Input: part model. Units: mm. Frame: model coordinates. Face numbers are marked on the shaded views. Coordinates: 2 decimals unless noted, no trailing zeros. Write each loop counter-clockwise with the first axis right and the second up, starting at its lowest first coordinate (ties: lowest second). Pieces come first, ordered by that corner, then holes. Notation, with made-up numbers: (74, 31) - (128, 31) arc R19 ccw to (128, 41) - close; hole circle Ø7 at (-10, -10.5). An arc over 180 degrees is marked (long way). Use CSV: the item, a comma, the result in double quotes.
```python
from build123d import *

# Parameters (mm, degrees)
SKETCH1_R           = 12.4
BOSS_EXTRUDE1_DEPTH = 59
SKETCH2_R           = 1.5
CUT_EXTRUDE1_DEPTH  = 3.4798
SKETCH4_R           = 4
BOSS_EXTRUDE3_DEPTH = 2.3
SKETCH5_R           = 2
BOSS_EXTRUDE4_DEPTH = 15.5


with BuildPart() as part:
    # Sketch1 → Boss-Extrude1 (new body)
    with BuildSketch(Plane(origin=(0, 0, 0), x_dir=(1, 0, 0), z_dir=(0, 1, 0))):
        with Locations(Location((0, 0, 0), (0, 0, 90))):
            Circle(SKETCH1_R)
    extrude(amount=BOSS_EXTRUDE1_DEPTH)

    # Sketch2 → Cut-Extrude1 (cut)
    with BuildSketch(Plane(origin=(0, 59, 0), x_dir=(1, 0, 0), z_dir=(0, 1, 0))):
        with Locations(Location((0, 8.5, 0), (0, 0, 270))):
            Circle(SKETCH2_R)
        with Locations(Location((0, -8.5, 0), (0, 0, 270))):
            Circle(SKETCH2_R)
    extrude(amount=-CUT_EXTRUDE1_DEPTH, mode=Mode.SUBTRACT)

    # Sketch4 → Boss-Extrude3 (add)
    with BuildSketch(Plane(origin=(0, 59, 0), x_dir=(1, 0, 0), z_dir=(0, 1, 0))):
        with Locations(Location((0, 0, 0), (0, 0, 270))):
            Circle(SKETCH4_R)
    extrude(amount=BOSS_EXTRUDE3_DEPTH)

    # Sketch5 → Boss-Extrude4 (add)
    with BuildSketch(Plane(origin=(0, 61.3, 0), x_dir=(1, 0, 0), z_dir=(0, 1, 0))):
        with Locations(Location((0, 0, 0), (0, 0, 270))):
            Circle(SKETCH5_R)
    extrude(amount=BOSS_EXTRUDE4_DEPTH)


solid = part.part
```
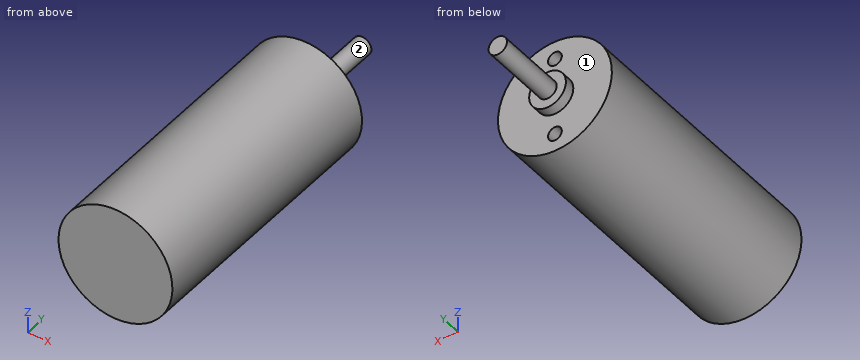
(1) Cut plane B-B on y = 30. Return loops of the section in (x, z), and give its area (3 significant figures).
Check values:
outline,"circle Ø24.8 at (0, 0)"
area,"483 mm^2"
(2) Draft query along Z for the marked faces 1 and 2. Return one class per face: pulls with the +Z half, pulls with the -Z half, needs draft (parallel to the pull), parting line crosses it, or undercut.
Check values:
face 1,"needs draft"
face 2,"parting line crosses it"
(3) Ray query, probe 1 along Y at (x, z) = (8.25, 2); probe 2 along Y at (x, z) = (2.25, 0); probe 3 along X at (y, z) = (20, -5.75). Return the intervals inside material, ascending. Write a range as from..to.
Check values:
probe 1,"0..59"
probe 2,"0..61.3"
probe 3,"-10.99..10.99"
(4) Pin query (flat end, axial travel): pin 1 Ø3 at (x, y) = (7, 55) entering from -Z; pin 2 Ø6 at (x, y) = (-9, 30.5) entering from +Z; pin 3 Ø3.5 at (x, z) = (0.5, -8) entering from +Y. Return the tip coordinate at first contact, or that it passes through.
Check values:
pin 1,"z = -11.11"
pin 2,"z = 10.85"
pin 3,"y = 59"
(5) Cut plane D-D on z = -9. Return loops of the section in (x, y), and give its area (3 significant figures).
Check values:
outline,"(-8.53, 0) - (8.53, 0) - (8.53, 59) - (1.41, 59) - (1.41, 55.52) - (-1.41, 55.52) - (-1.41, 59) - (-8.53, 59) - close"
area,"997 mm^2"
(6) Cut plane A-A on z = 0. Return loops of the section in (x, y).
Check values:
outline,"(-12.4, 0) - (12.4, 0) - (12.4, 59) - (4, 59) - (4, 61.3) - (2, 61.3) - (2, 76.8) - (-2, 76.8) - (-2, 61.3) - (-4, 61.3) - (-4, 59) - (-12.4, 59) - close"
(7) Cut plane C-C on x = 3.25. Return loops of the section in (y, z), and give its area (3 significant figures).
Check values:
outline,"(0, -11.97) - (59, -11.97) - (59, -2.33) - (61.3, -2.33) - (61.3, 2.33) - (59, 2.33) - (59, 11.97) - (0, 11.97) - close"
area,"1,420 mm^2"
